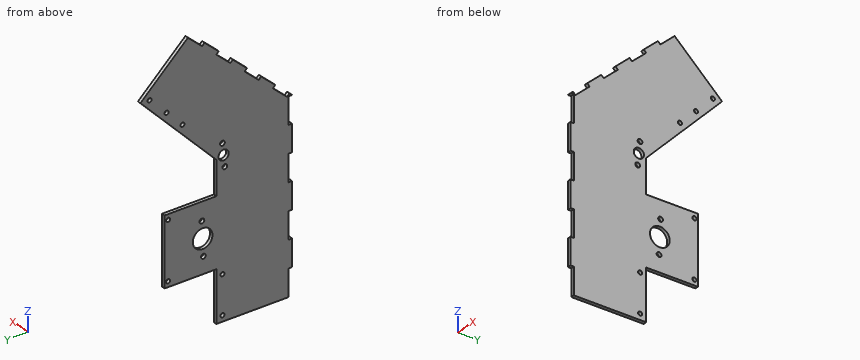
```python
from build123d import *

# Parameters (mm, degrees)
SKETCH1_R           = 1.75
SKETCH1_R_2         = 3.75
SKETCH1_R_3         = 7.25
BOSS_EXTRUDE1_DEPTH = 2.5
SKETCH2_R           = 1.5
CUT_EXTRUDE1_DEPTH  = 45.72
SKETCH3_W           = 19.957142857
SKETCH3_H           = 2.5
CUT_EXTRUDE2_DEPTH  = 2.54
CUT_EXTRUDE3_DEPTH  = 2.54


with BuildPart() as part:
    # Sketch1 → Boss-Extrude1 (new body)
    with BuildSketch(Plane(origin=(0, 0, 0), x_dir=(0, 0, -1), z_dir=(1, 0, 0))):
        Polygon((0, 0), (25.4, 0), (25.4, 38.1), (76.2, 38.1), (76.2, 0), (114.3, 0), (114.3, -55.88), (-25.4, -55.88), (-93.919230144, 19.137831884), (-58.936151167, 55.972926363), align=None)
        with Locations((-9.840865869, -4.523881045)):
            Circle(SKETCH1_R, mode=Mode.SUBTRACT)
        with Locations((-1.386257564, -5.40114863)):
            Circle(SKETCH1_R_2, mode=Mode.SUBTRACT)
        with Locations((7.06835074, -6.278416216)):
            Circle(SKETCH1_R, mode=Mode.SUBTRACT)
        with Locations((51.390541055, 10.062014111)):
            Circle(SKETCH1_R_3, mode=Mode.SUBTRACT)
        with Locations((38.902844079, 10.616472631)):
            Circle(SKETCH1_R, mode=Mode.SUBTRACT)
        with Locations((63.87823803, 9.507555591)):
            Circle(SKETCH1_R, mode=Mode.SUBTRACT)
    extrude(amount=BOSS_EXTRUDE1_DEPTH)

    # Sketch2 → Cut-Extrude1 (cut)
    with BuildSketch(Plane.ZY):
        with Locations((-72.089288217, 35.554137698)):
            Circle(SKETCH2_R)
        with Locations((-29.434072146, 35.554137698)):
            Circle(SKETCH2_R)
        with Locations((-109.810505414, -4.492241592)):
            Circle(SKETCH2_R)
        with Locations((-81.28, -4.492241592)):
            Circle(SKETCH2_R)
        with Locations((58.584658566, 49.213818775)):
            Circle(SKETCH2_R)
        with Locations((45.481260754, 36.702251461)):
            Circle(SKETCH2_R)
        with Locations((33.116955359, 24.896394578)):
            Circle(SKETCH2_R)
    extrude(amount=-CUT_EXTRUDE1_DEPTH, mode=Mode.SUBTRACT)

    # Sketch3 → Cut-Extrude2 (cut)
    with BuildSketch(Plane.ZY):
        with Locations((-104.321428572, -54.63)):
            Rectangle(SKETCH3_W, SKETCH3_H)
        with Locations((-64.407142858, -54.63)):
            Rectangle(SKETCH3_W, SKETCH3_H)
        with Locations((-24.492857143, -54.63)):
            Rectangle(SKETCH3_W, SKETCH3_H)
        with Locations((15.421428572, -54.63)):
            Rectangle(SKETCH3_W, SKETCH3_H)
    extrude(amount=-CUT_EXTRUDE2_DEPTH, mode=Mode.SUBTRACT)

    # Sketch4 → Cut-Extrude3 (cut)
    with BuildSketch(Plane.ZY):
        Polygon((27.232932154, -53.873226195), (36.759546153, -43.443075041), (34.913634935, -41.757070362), (25.387020937, -52.187221516), align=None)
        Polygon((44.440248934, -31.326919208), (46.286160151, -33.012923887), (55.81277415, -22.582772733), (53.966862932, -20.896768054), align=None)
        Polygon((63.493476931, -10.4666169), (65.339388148, -12.152621579), (74.866002147, -1.722470425), (73.020090929, -0.036465746), align=None)
        Polygon((82.546704928, 10.393685408), (84.392616145, 8.70768073), (93.919230144, 19.137831884), (92.193270327, 20.955164571), align=None)
    extrude(amount=-CUT_EXTRUDE3_DEPTH, mode=Mode.SUBTRACT)


solid = part.part
```
Read the model definition and answer for the solid it produces. Units are mm, in the model's axes. Give positions to 0.01 mm unless a question says otherwise; leave off trailing zeros. Order: outer loops, then holes, each group sorted by start corner. A loop starts at its lowest first (then second) coordinate and runs counter-clockwise, first axis right, second up.
(1) Find section A-A (z = -50). Give the vertices of the cut face in (x, y).
(2) Find section B-B (z = -91.5). Give the vertices of the cut face in (x, y), plus the area to 3 significant figures.
(3) Given pin 1 (1.2 mm diameter, centred on x = 1.5, y = -55, fed in from -Z); pin 2 (4.5 mm diameter, centred on y = -5.4, z = 1.39, fed in from +X); pin 3 (1.2 mm diameter, centred on x = 1, y = 23.5, fed in from +Z); pin 4 (1.5 mm diameter, centred on x = 1, y = -7, fed in from +Z), each flat-ended and moving along its own axis, determine where each tip first touches the part or whether it passes through.
(4) Find section D-D (y = 42). Give the vertices of the cut face in (x, z).
(5) Find section C-C (x = 1.3). Give the number of separate pieces and of enclosed holes in the cut face, plus the area to 3 significant figures.
(6) Straight lines are drawn through the part: L1, parallel to Z at x = 0.85, y = -5; L2, parallel to Z at x = 2, y = 11; L3, parallel to Y at x = 1.8, z = -81. For each, find the intervals that lie inside material, in ascending order.
Result sheet:
1. outline: (0, -55.88) - (2.5, -55.88) - (2.5, 2.95) - (0, 2.95) - close; (0, 17.18) - (2.5, 17.18) - (2.5, 38.1) - (0, 38.1) - close
2. outline: (0, -55.88) - (2.5, -55.88) - (2.5, 0) - (0, 0) - close
2. area: 140 mm2
3. pin 1: stops at z = -94.34
3. pin 2: passes through
3. pin 3: stops at z = 90.35
3. pin 4: stops at z = 67.34
4. outline: (0, 44.22) - (2.5, 44.22) - (2.5, 72.21) - (0, 72.21) - close
5. separate pieces: 1
5. enclosed holes: 13
5. area: 13,300 mm2
6. L1: z = -114.3 to -111.22, -108.4 to -82.69, -79.87 to -8.26, -5.87 to -2.34, 5.11 to 8.16, 11.52 to 68.49
6. L2: z = -76.2 to -64.79, -62.96 to -58.58, -44.2 to -40.61, -37.2 to -25.4, 11.58 to 83.1
6. L3: y = -55.88 to -5.97, -3.02 to 0
